Geometry: final body of the model. Coordinates: model frame, mm. Face numbers are marked on the shaded views. A direction names the side the tool comes from. Round coordinates to 2 decimals unless told otherwise and drop trailing zeros. Write each loop counter-clockwise with the first axis right and the second up, starting at its lowest first coordinate (ties: lowest second). Pieces come first, ordered by that corner, then holes. Notation, with made-up numbers: M 82,-23 L 137,-23 A37 ccw 137,15 Z; hole C 1.25,17.5 d7. An arc over 180 degrees is marked long. Answer as CSV lines item,"result". Start each with the question number.
Q1. First-contact query: pin 1 (4 mm diameter, centred on x = 1, z = 6, fed in from +Y). Flat tip, straight axial feed; report the tip coordinate or a pass-through.
Q2. Ray query, probe 1 along Y at (x, z) = (0, 0.85); probe 2 along Z at (x, y) = (1.25, 4); probe 3 along Y at (x, z) = (-3, 13.5). Return the intervals inside material, ascending.
Q3. Reachability of the marked faces 1 and 2 from +Z, -Z, +X, -X, +Y, -Y: full face, straight path, thin tool, end or side. Return the list, or none.
Q4. Section query C-C on z = 10. Output: boundary loops of the cut face in (x, y), and give its area (3 significant figures).
Q5. Section query D-D on z = 2.75. Output: boundary loops of the cut face in (x, y), and give its area (3 significant figures).
Q6. Section query A-A on x = 0. Output: boundary loops of the cut face in (y, z), and give its area (3 significant figures).
Q7. Section query B-B on y = 8.5. Output: boundary loops of the cut face in (x, z).
Q8. Mould query, pull axis X, two halves, no side actions, for the marked faces 3, 4, 5 and 6. Classes: pulls with the +X half, pulls with the -X half, needs draft (parallel to the pull), parting line crosses it, or undercut.
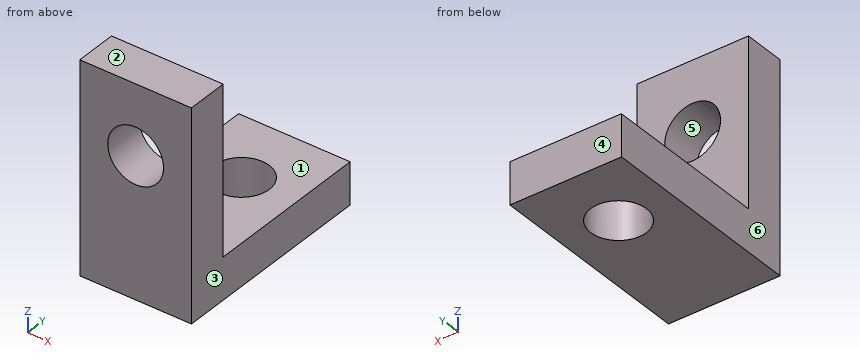
```python
from build123d import *

# Parameters (mm, degrees)
ESQUISSE1_W             = 8
ESQUISSE1_H             = 3
BOSS_EXTRU_1_DEPTH      = 15
ESQUISSE2_W             = 8
ESQUISSE2_H             = 3
BOSS_EXTRU_2_DEPTH      = 12
ESQUISSE3_R             = 2
ENL_V_MAT_EXTRU_1_DEPTH = 20.62141687
ESQUISSE4_R             = 2
ENL_V_MAT_EXTRU_2_DEPTH = 19.5


with BuildPart() as part:
    # Esquisse1 → Boss.-Extru.1 (new body)
    with BuildSketch(Plane.XY):
        Rectangle(ESQUISSE1_W, ESQUISSE1_H)
    extrude(amount=BOSS_EXTRU_1_DEPTH)

    # Esquisse2 → Boss.-Extru.2 (add)
    with BuildSketch(Plane(origin=(0, 1.5, 0), x_dir=(1, 0, 0), z_dir=(0, 1, 0))):
        with Locations((0, -1.5)):
            Rectangle(ESQUISSE2_W, ESQUISSE2_H)
    extrude(amount=BOSS_EXTRU_2_DEPTH)

    # Esquisse3 → Enlèv. mat.-Extru.1 (cut, through all)
    with BuildSketch(Plane(origin=(0, 1.5, 0), x_dir=(1, 0, 0), z_dir=(0, 1, 0))):
        with Locations(Location((0, -10, 0), (0, 0, 270))):
            Circle(ESQUISSE3_R)
    extrude(amount=-ENL_V_MAT_EXTRU_1_DEPTH, mode=Mode.SUBTRACT)

    # Esquisse4 → Enlèv. mat.-Extru.2 (cut, through all)
    with BuildSketch(Plane.XY.offset(3)):
        with Locations((0, 8.5)):
            Circle(ESQUISSE4_R)
    extrude(amount=-ENL_V_MAT_EXTRU_2_DEPTH, mode=Mode.SUBTRACT)


solid = part.part
```
Entries:
1,pin 1,"stops at y = 1.5"
2,probe 1,"y = -1.5 to 6.5, 10.5 to 13.5"
2,probe 2,"z = 0 to 3"
2,probe 3,"y = -1.5 to 1.5"
3,face 1,"+Z, +X, -X, +Y"
3,face 2,"+Z, +X, -X, +Y, -Y"
4,outline,"M -4,-1.5 L -2,-1.5 L -2,1.5 L -4,1.5 Z; M 2,-1.5 L 4,-1.5 L 4,1.5 L 2,1.5 Z"
4,area,"12.0 mm^2"
5,outline,"M -4,-1.5 L 4,-1.5 L 4,13.5 L -4,13.5 Z; hole C 0,8.5 d4"
5,area,"107 mm^2"
6,outline,"M -1.5,0 L 6.5,0 L 6.5,3 L 1.5,3 L 1.5,8 L -1.5,8 Z; M -1.5,12 L 1.5,12 L 1.5,15 L -1.5,15 Z; M 10.5,0 L 13.5,0 L 13.5,3 L 10.5,3 Z"
6,area,"57.0 mm^2"
7,outline,"M -4,0 L -2,0 L -2,3 L -4,3 Z; M 2,0 L 4,0 L 4,3 L 2,3 Z"
8,face 3,"pulls with the +X half"
8,face 4,"needs draft"
8,face 5,"undercut"
8,face 6,"pulls with the -X half"
